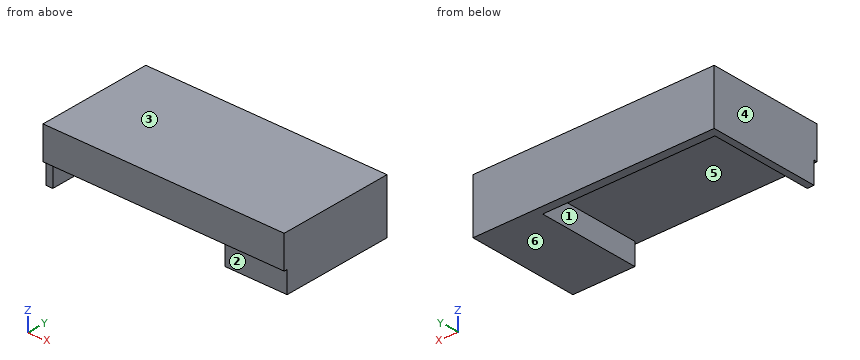
from build123d import *

# Parameters (mm, degrees)
F0_W     = 140
F0_H     = 31.75
F1_DEPTH = 66.9
F3_DEPTH = 12.7


with BuildPart() as f1:
    # F0 (on Front) → F1 (new body)
    with BuildSketch(Plane.XZ):
        with Locations((70, 15.875)):
            Rectangle(F0_W, F0_H)
    extrude(amount=F1_DEPTH)

    # F2 (on face) → F3 (cut)
    with BuildSketch(Plane(origin=(0, 0, 0), x_dir=(1, 0, 0), z_dir=(0, 0, -1))):
        Polygon((0, 66.9), (0, 65), (4, 65), (4, 5), (104, 5), (104, 65), (140, 65), (140, 66.9), align=None)
    extrude(amount=-F3_DEPTH, mode=Mode.SUBTRACT)


solid = f1.part
Source: CAD feature listing. Evaluate the final solid. Frame: model axes, mm. Face numbers are marked on the shaded views. A direction names the side the tool comes from. Round coordinates to 2 decimals unless told otherwise and drop trailing zeros. Write each loop counter-clockwise with the first axis right and the second up, starting at its lowest first coordinate (ties: lowest second). Pieces come first, ordered by that corner, then holes. Notation, with made-up numbers: M -29,88.5 L -1,88.5 A14 ccw -1,109.5 Z; hole C -37.5,25 d10. An arc over 180 degrees is marked long. One line per item, written item: value. Start each with the question number.
Item 1: Pin query (flat end, axial travel): pin 1 (10 mm diameter, centred on x = 119.5, z = 7.5, fed in from -Y); pin 2 (12 mm diameter, centred on x = 97, y = -55, fed in from -Z). Return the tip coordinate at first contact, or that it passes through.
Item 2: Section query A-A (y = -32). Return the cut outline in (x, z), plus the area to 4 significant figures.
Item 3: Set-up query: the marked faces 1, 2 and 3. Return all of +Z, -Z, +X, -X, +Y, -Y with unobstructed straight access to the full face (end or side cutting, diameter ignored); none if empty.
Item 4: Section query B-B (x = 67.5). Return the cut outline in (y, z), plus the area to 3 significant figures.
Item 5: Ray query, L1, parallel to X at y = -21, z = 4; L2, parallel to Z at x = 60.5, y = -23; L3, parallel to Y at x = 58, z = 9. Return the intervals inside material, ascending. Write a range as from..to.
Item 6: Mould query, pull axis X, two halves, no side actions, for the marked faces 4, 5 and 6. Classes: pulls with the +X half, pulls with the -X half, needs draft (parallel to the pull), parting line crosses it, or undercut.
Result set:
1. pin 1: stops at y = -65
1. pin 2: stops at z = 12.7
2. outline: M 0,0 L 4,0 L 4,12.7 L 104,12.7 L 104,0 L 140,0 L 140,31.75 L 0,31.75 Z
2. area: 3,175 mm²
3. face 1: -Z, -Y
3. face 2: -Z, +X, -X, -Y
3. face 3: +Z, +X, -X, +Y, -Y
4. outline: M -66.9,12.7 L -5,12.7 L -5,0 L 0,0 L 0,31.75 L -66.9,31.75 Z
4. area: 1,340 mm²
5. L1: x = 0..4, 104..140
5. L2: z = 12.7..31.75
5. L3: y = -5..0
6. face 4: pulls with the -X half
6. face 5: undercut
6. face 6: needs draft
